Design review of the part built by this model. Coordinates are the model's own, in mm. Round coordinates to 2 decimals unless told otherwise and drop trailing zeros. Order: outer loops, then holes, each group sorted by start corner. A loop starts at its lowest first (then second) coordinate and runs counter-clockwise, first axis right, second up.
from build123d import *

# Parameters (mm, degrees)
SKETCH1_W           = 160
SKETCH1_H           = 110
BOSS_EXTRUDE1_DEPTH = 5
SKETCH3_W           = 152
SKETCH3_H           = 102
CUT_EXTRUDE1_DEPTH  = 1.6
SKETCH4_R           = 1.4
BOSS_EXTRUDE3_DEPTH = 2.5
SKETCH11_W          = 5
SKETCH11_H          = 40
CUT_EXTRUDE3_DEPTH  = 1.6


with BuildPart() as part:
    # Sketch1 → Boss-Extrude1 (new body)
    with BuildSketch(Plane(origin=(0, 0, 0), x_dir=(1, 0, 0), z_dir=(0, 0, -1))):
        with Locations((80, 55)):
            Rectangle(SKETCH1_W, SKETCH1_H)
    extrude(amount=-BOSS_EXTRUDE1_DEPTH)

    # Sketch3 → Cut-Extrude1 (cut)
    with BuildSketch(Plane(origin=(0, 0, 5), x_dir=(-1, 0, 0), z_dir=(0, 0, 1))):
        with Locations((-80, 55)):
            Rectangle(SKETCH3_W, SKETCH3_H)
    extrude(amount=-CUT_EXTRUDE1_DEPTH, mode=Mode.SUBTRACT)

    # Sketch4 → Boss-Extrude3 (add)
    with BuildSketch(Plane(origin=(0, 0, 3.4), x_dir=(-1, 0, 0), z_dir=(0, 0, 1))):
        with Locations((-152, 102)):
            Circle(SKETCH4_R)
        with Locations((-8, 102)):
            Circle(SKETCH4_R)
        with Locations((-152, 8)):
            Circle(SKETCH4_R)
        with Locations((-8, 8)):
            Circle(SKETCH4_R)
    extrude(amount=BOSS_EXTRUDE3_DEPTH)

    # Sketch11 → Cut-Extrude3 (cut)
    with BuildSketch(Plane(origin=(0, 0, 5), x_dir=(-1, 0, 0), z_dir=(0, 0, 1))):
        with Locations((-158.5, 55)):
            Rectangle(SKETCH11_W, SKETCH11_H)
        with Locations((-1.5, 55)):
            Rectangle(SKETCH11_W, SKETCH11_H)
    extrude(amount=-CUT_EXTRUDE3_DEPTH, mode=Mode.SUBTRACT)


solid = part.part
1) Clearance check with a flat-ended pin moving along its axis: P1, Ø1.5, axis at x = 130, y = -71, coming from the +Z side. State where the tip first meets the part, or that it passes through.
Results:
P1: stops at z = 3.4
2) Take a section at A-A on x = 127. Give the boundary of the cut face in (y, z), plus the area to 3 significant figures.
Results:
outline: (-110, 0) - (0, 0) - (0, 5) - (-4, 5) - (-4, 3.4) - (-106, 3.4) - (-106, 5) - (-110, 5) - close
area: 387 mm2
3) The part is to be moulded in two halves that separate along Y. For faces 1 (the face through (80, -107, 5)), 2 (the face through (79, 0, 2)), 3 (the face through (81, -56, 3.4)), say which applies: released by +Y, released by -Y, zero draft, split by the parting line, or undercut.
Results:
face 1: zero draft
face 2: released by +Y
face 3: undercut
4) Take a section at B-B on y = -17. Give the boundary of the cut face in (x, z), plus the area to 3 significant figures.
Results:
outline: (0, 0) - (160, 0) - (160, 5) - (156, 5) - (156, 3.4) - (4, 3.4) - (4, 5) - (0, 5) - close
area: 557 mm2
5) To check wall thickness, follow line 1 along Y through (x, z) = (23, 3.65); line 2 along X through (y, z) = (-93, 4.5); line 3 along Z through (x, y) = (127.5, -103). State the ranges of each line that lie inside material, in increasing order.
Results:
line 1: y = -110 to -106, -4 to 0
line 2: x = 0 to 4, 156 to 160
line 3: z = 0 to 3.4
